Autodesk Inventor part; units mm, degrees
ref_plane "YZ Plane" through (0, 0, 0) normal (1, 0, 0) x (0, 1, 0)
ref_plane "XZ Plane" through (0, 0, 0) normal (0, 1, 0) x (-1, 0, 0)
ref_plane "XY Plane" through (0, 0, 0) normal (0, 0, 1) x (1, 0, 0)
sketch "Sketch1" plane through (0, 0, 0) normal (0, 0, 1) x (1, 0, 0)
  line L0 (-6.3366, 6.9163) -> (21.6034, 6.9163)
  line L1 (21.6034, 6.9163) -> (21.6034, -8.3237)
  line L2 (21.6034, -8.3237) -> (-6.3366, -8.3237)
  line L3 (-6.3366, -8.3237) -> (-6.3366, 6.9163)
  point P0 (0, 0)
  dimension "d0" = 27.94
  dimension "d1" = 15.24
extrude "Extrusion1" add sketch "Sketch1" along normal blind 7.62
sketch "Sketch2" plane through (0, 0, 7.62) normal (0, 0, 1) x (1, 0, 0)
  line L0 (-6.3366, 6.9163) -> (-6.3366, -8.3237)
  line L1 (21.6034, -8.3237) -> (21.6034, 6.9163)
  line L2 (21.6034, 0.3123) -> (21.6034, 2.7253)
  line L3 (-6.3366, 2.7253) -> (-6.3366, 0.3123)
  line L4 (21.6034, 6.9163) -> (-6.3366, 6.9163)
  line L5 (-6.3366, -8.3237) -> (21.6034, -8.3237)
  line L6 (0.9631, 2.7253) -> (-0.2406, 2.7253)
  line L7 (-0.2406, 0.3123) -> (0.9631, 0.3123)
  line L8 (-0.2406, 0.3123) -> (-0.2406, 2.7253)
  line L9 (-0.2406, 0.3123) -> (3.0821, 0.3123)
  line L10 (3.0821, 0.3123) -> (3.0821, 2.7253)
  line L11 (3.0821, 2.7253) -> (-0.2406, 2.7253)
  line L12 (-0.2406, 2.7253) -> (-0.2406, 0.3123)
  line L13 (14.3038, 2.7253) -> (15.5074, 2.7253)
  line L14 (15.5074, 0.3123) -> (14.3038, 0.3123)
  line L15 (15.5074, 0.3123) -> (15.5074, 2.7253)
  line L16 (15.5074, 0.3123) -> (12.1847, 0.3123)
  line L17 (12.1847, 0.3123) -> (12.1847, 2.7253)
  line L18 (12.1847, 2.7253) -> (15.5074, 2.7253)
  line L19 (15.5074, 2.7253) -> (15.5074, 0.3123)
  line L20 (-6.3366, -0.7037) -> (21.6034, -0.7037)
  line L21 (-6.3366, 2.7253) -> (21.6034, 2.7253)
  line L22 (21.6034, 2.7253) -> (21.6034, 0.3123)
  line L23 (21.6034, 0.3123) -> (-6.3366, 0.3123)
  line L24 (-6.3366, 0.3123) -> (-6.3366, 2.7253)
  point P0 (0, 0)
  point P1 (-0.2406, 1.5188)
  point P2 (15.2669, 0)
  point P3 (15.5074, 1.5188)
  dimension "d6" = 6.096
extrude "Extrusion2" add sketch "Sketch2" along normal blind 8.7376 contours L6 L11 L10 L9 L7 L8 | L15 L14 L16 L17 L18 L13
sketch "Sketch3" plane through (-0.2406, 2.7253, 7.62) normal (0, 1, 0) x (1, 0, 0)
  line L0 (3.3227, -8.7376) -> (0, -8.7376)
  line L1 (3.3227, -8.7376) -> (0, -8.7376)
  line L2 (-6.096, 7.62) -> (21.844, 7.62)
  line L3 (3.3227, -11.3552) -> (3.3227, -8.7376)
  line L4 (12.4253, -8.7376) -> (15.748, -8.7376)
  line L5 (12.4253, -8.7376) -> (15.748, -8.7376)
  line L6 (12.4253, -11.3552) -> (12.4253, -8.7376)
  line L7 (15.748, -8.7376) -> (17.2091, -8.255)
  line L8 (17.2091, -8.255) -> (17.2091, -15.2732)
  line L9 (17.2091, -15.2732) -> (14.9854, -19.057)
  line L10 (14.9854, -19.057) -> (12.4253, -19.057)
  line L11 (12.4253, -19.057) -> (12.4253, -8.7376)
  line L12 (7.874, 7.62) -> (7.874, -24.8322)
  line L13 (3.3227, -8.7376) -> (0, -8.7376)
  line L14 (3.3227, -8.7376) -> (0, -8.7376)
  line L15 (3.3227, -11.3552) -> (3.3227, -8.7376)
  line L16 (0, -8.7376) -> (-1.4611, -8.255)
  line L17 (-1.4611, -8.255) -> (-1.4611, -15.2732)
  line L18 (-1.4611, -15.2732) -> (0.7626, -19.057)
  line L19 (0.7626, -19.057) -> (3.3227, -19.057)
  line L20 (3.3227, -19.057) -> (3.3227, -8.7376)
  point P0 (0.2406, 7.62)
extrude "Extrusion4" add sketch "Sketch2" along normal blind 25.4 contours L6 L11 L10 L9 L7 L8 | L15 L14 L16 L17 L18 L13
sketch "Sketch4" plane through (-6.3366, 6.9163, 0) normal (0, 1, 0) x (1, 0, 0)
  point P0 (6.3366, 0)
sketch "Sketch5" plane through (0, 0, 7.62) normal (0, 0, 1) x (1, 0, 0)
  line L0 (21.6034, 6.9163) -> (-6.3366, 6.9163)
  line L1 (-6.3366, 15.6735) -> (21.6034, 15.6735)
  line L2 (21.6034, 15.6735) -> (21.6034, 6.9163)
  line L3 (21.6034, 6.9163) -> (-6.3366, 6.9163)
  line L4 (-6.3366, 6.9163) -> (-6.3366, 15.6735)
  point P0 (0, 0)
extrude "Extrusion5" add sketch "Sketch5" along normal blind 17.145 and the other way blind 7.62
extrude "Extrusion6" cut sketch "Sketch2" against normal blind 25.4 contours L20 L1 L5 L0
extrude "Extrusion7" add sketch "Sketch2" along normal blind 4.7625 contours L21 L8 L23 L0 | L1 L23 L15 L21 | L21 L17 L23 L10
extrude "Extrusion8" add sketch "Sketch3" against normal up to surface (2.413 mm away)
sketch "Sketch6" plane through (-6.3366, 0.3123, 7.62) normal (0, -1, 0) x (1, 0, 0)
  line L0 (27.94, 0) -> (27.94, 4.7625)
  line L1 (21.844, 4.7625) -> (21.844, 8.7376)
  line L2 (27.94, 0) -> (21.844, 0)
  line L3 (21.844, 0) -> (21.844, 4.7625)
  line L4 (21.844, 4.7625) -> (27.94, 4.7625)
  line L5 (27.94, 4.7625) -> (27.94, 0)
  line L6 (18.5213, 4.7625) -> (18.5213, 25.4)
  line L7 (18.5213, 4.7625) -> (9.4187, 4.7625)
  line L8 (9.4187, 4.7625) -> (9.4187, 0)
  line L9 (9.4187, 0) -> (18.5213, 0)
  line L10 (18.5213, 0) -> (18.5213, 4.7625)
  line L11 (6.096, 4.7625) -> (6.096, 8.7376)
  line L12 (0, 0) -> (0, 4.7625)
  line L13 (6.096, 4.7625) -> (0, 4.7625)
  line L14 (0, 4.7625) -> (0, 0)
  line L15 (0, 0) -> (6.096, 0)
  line L16 (6.096, 0) -> (6.096, 4.7625)
  point P0 (6.3366, -7.62)
  point P1 (18.5213, 19.057)
extrude "Extrusion9" cut sketch "Sketch6" against normal up to surface (6.604 mm away)
sketch "Sketch7" plane through (12.1847, 0.3123, 7.62) normal (0, -1, 0) x (1, 0, 0)
  line L0 (3.3227, 17.7594) -> (4.7838, 15.2732)
  line L1 (3.3227, 17.7594) -> (2.3659, 19.3874)
  line L2 (2.3659, 19.3874) -> (2.3659, 25.4)
  line L3 (3.3227, 25.4) -> (0, 25.4)
  line L4 (3.3227, 17.7594) -> (3.3227, 25.4)
  line L5 (2.3659, 25.4) -> (3.3227, 25.4)
  line L6 (3.3227, 25.4) -> (3.3227, 17.7594)
  line L7 (-18.5213, -7.62) -> (9.4187, -7.62)
  line L8 (-12.4253, 17.7594) -> (-11.4685, 19.3874)
  line L9 (-11.4685, 19.3874) -> (-11.4685, 25.4)
  line L10 (-12.4253, 17.7594) -> (-12.4253, 25.4)
  line L11 (-11.4685, 25.4) -> (-12.4253, 25.4)
  line L12 (-12.4253, 25.4) -> (-12.4253, 17.7594)
  point P0 (-12.1847, -7.62)
extrude "Extrusion10" cut sketch "Sketch7" against normal up to surface (6.604 mm away)
fillet "Fillet1" radius 3.175 4 edges at (0.7162, 1.5188, 33.02) (14.5507, 1.5188, 33.02) (16.9686, 1.5188, 22.8932) (-1.7017, 1.5188, 22.8932)
properties part number "Attachment1"
Geometry check sheet. Reference: the model listing, model coordinates, mm. A direction names the side the tool comes from. Give positions to 0.01 mm unless a question says otherwise; leave off trailing zeros. Loops run counter-clockwise (first coordinate to the right, second up) from the corner with the lowest first, then second, coordinate; pieces in that order, holes last. Notation, with made-up numbers: M 35.5,67.5 L 70.5,67.5 A24 cw 70.5,97.5 Z; hole C -17,43.25 d4. An arc over 180 degrees is marked long. Answer as a JSON object with one key per item and string values. Group by question number.
Item 1: Sectioned sample at B-B on z = 18. Record the boundary of the cut face in (x, y).
Item 2: Access from +Z, -Z, +X, -X, +Y, -Y to the whole of each face (thin tool, end or side, straight path). Record for faces 4 (the flat face through (0.716, 2, 28)), 5 (the cylindrical face through (16.854, 1.536, 22.874)), 6 (the cylindrical face through (-1.593, 1.536, 22.851)), 7 (the flat face through (3.082, 2, 20)), 8 (the flat face through (8, 6.916, 16)).
Item 3: Gauge pin test, flat ends, axial feed: pin 1 (1.2 mm diameter, centred on y = 1.5, z = 18, fed in from -X); pin 2 (1.2 mm diameter, centred on y = 1.5, z = 26, fed in from -X); pin 3 (2.5 mm diameter, centred on y = 2, z = 29, fed in from +X). Record the tip position at first contact, or that the pin passes through.
Item 4: Material ranges on L1, parallel to X at y = 0.5, z = 11; L2, parallel to Y at x = 1.75, z = 19; L3, parallel to Y at x = 4.5, z = 22, recorded low to high.
Item 5: Mould release check, pull along X, two halves, no side actions. Record for faces 1 (the flat face through (12.185, 2, 20)), 2 (the flat face through (14.551, 2, 28)), 3 (the flat face through (-1.702, 2, 19)): pulls with the +X half, pulls with the -X half, needs draft (parallel to the pull), parting line crosses it, or undercut.
Item 6: Sectioned sample at D-D on z = 13. Record the boundary of the cut face in (x, y).
Item 7: Sectioned sample at A-A on z = 27.5. Record the boundary of the cut face in (x, y).
Findings below:
{
 "1": {"outline": "M -6.34,6.92 L 21.6,6.92 L 21.6,15.67 L -6.34,15.67 Z; M -1.7,0.31 L 3.08,0.31 L 3.08,2.73 L -1.7,2.73 Z; M 12.18,0.31 L 16.97,0.31 L 16.97,2.73 L 12.18,2.73 Z"},
 "2": {"face 4": "+Z, -X, +Y, -Y", "face 5": "+Z, +X, -Y", "face 6": "+Z, -X, -Y", "face 7": "+Z, -Y", "face 8": "+Z, +X, -X"},
 "3": {"pin 1": "x = -1.7", "pin 2": "x = -0.23", "pin 3": "x = 14.55"},
 "4": {"L1": "-0.24 to 3.08, 12.18 to 15.51", "L2": "0.31 to 2.73, 6.92 to 15.67", "L3": "6.92 to 15.67"},
 "5": {"face 1": "undercut", "face 2": "pulls with the +X half", "face 3": "pulls with the -X half"},
 "6": {"outline": "M -6.34,6.92 L 21.6,6.92 L 21.6,15.67 L -6.34,15.67 Z; M -0.24,0.31 L 3.08,0.31 L 3.08,2.73 L -0.24,2.73 Z; M 12.18,0.31 L 15.51,0.31 L 15.51,2.73 L 12.18,2.73 Z"},
 "7": {"outline": "M 0.72,0.31 L 3.08,0.31 L 3.08,2.73 L 0.72,2.73 Z; M 12.18,0.31 L 14.55,0.31 L 14.55,2.73 L 12.18,2.73 Z"}
}
